Source: three-view drawing plus pictorial views. Frame: mm from the lowest corner of the part. A direction names the side the tool comes from. Give positions to 0.01 mm unless a question says otherwise; leave off trailing zeros. Loops run counter-clockwise (first coordinate to the right, second up) from the corner with the lowest first, then second, coordinate; pieces in that order, holes last.
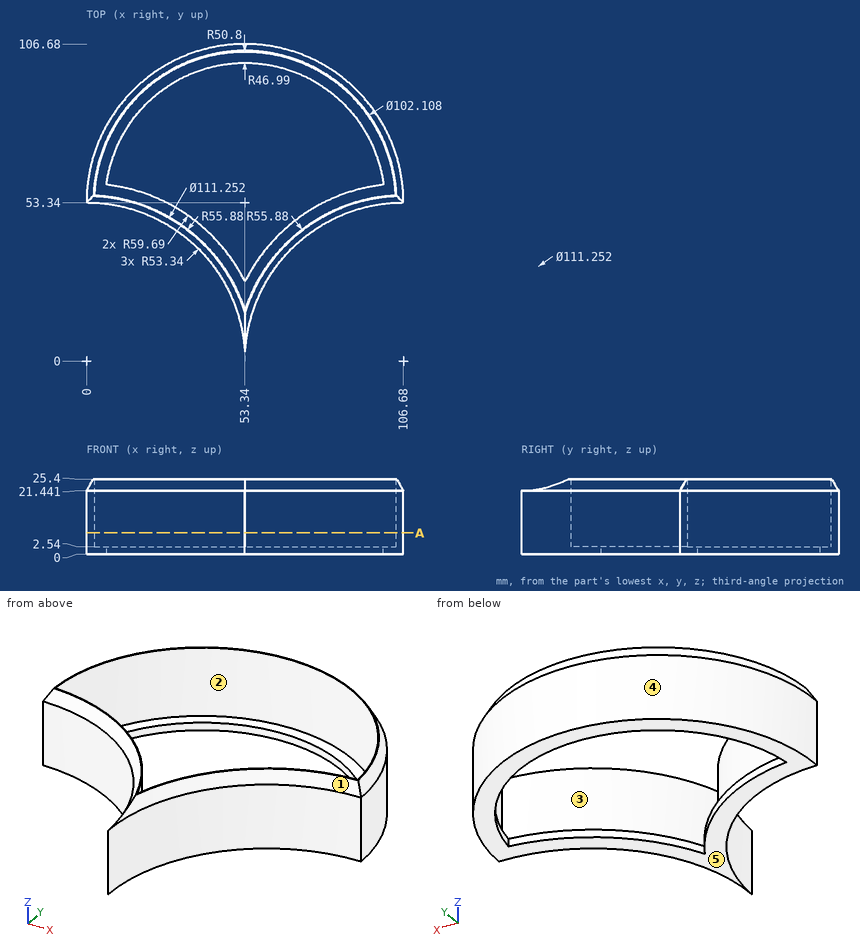
Q1. Material intervals for probe 1 along Y at (x, z) = (26, 19) (1 decimal); probe 2 along X at (y, z) = (41.5, 17.5); probe 3 along X at (y, z) = (75.5, 6.75), sorted ascending.
Q2. Mould query, pull axis Y, two halves, no side actions, for the marked faces 3, 4 and 5. Classes: +Y half, -Y half, draft (parallel to the pull), parting line (faces both ways), or undercut.
Q3. Reachability of the marked faces 1 and 2 from +Z, -Z, +X, -X, +Y, -Y: full face, straight path, thin tool, end or side. Return the list, or none.
Q4. Section query A-A, the plane z = 7.25. Return loops of the section in (x, y) (1 decimal).
Q5. Pin query (flat end, axial travel): pin 1 Ø8 at (y, z) = (32, 3.5) entering from -X; pin 2 Ø2 at (x, z) = (59.5, 17.5) entering from +Y; pin 3 Ø8 at (y, z) = (65, 8.5) entering from +X. Return the tip coordinate at first contact, or that it passes through.
Resolved:
1. probe 1: y = 46.6 to 49.5, 96.2 to 99.1
1. probe 2: x = 33.51 to 37.42, 69.26 to 73.17
1. probe 3: x = 4.82 to 7.63, 99.05 to 101.86
2. face 3: undercut
2. face 4: +Y half
2. face 5: draft
3. face 1: +Z, +X, -Y
3. face 2: +Z
4. outline: (0, 53.3) arc R53.3 cw to (53.3, 0) arc R53.3 cw to (106.7, 53.3) arc R53.3 ccw to start; hole (2.6, 55.8) arc R55.9 cw to (53.3, 16.7) arc R55.9 cw to (104.1, 55.8) arc R50.8 ccw to start
5. pin 1: stops at x = 39.36
5. pin 2: stops at y = 106.43
5. pin 3: stops at x = 106.13
